Part model, mm, in its own coordinate system. A direction names the side the tool comes from. Round coordinates to 2 decimals unless told otherwise and drop trailing zeros. Loops run counter-clockwise (first coordinate to the right, second up) from the corner with the lowest first, then second, coordinate; pieces in that order, holes last.
(1) Cut at D-D on x = -13.5. List the corners of the cut face in (y, z), then the cut area to 3 significant figures.
(2) Tool access for faces 5 (the face through (-41.03, -29.13, 3.86)), 6 (the face through (23.855, -29.125, 33.602)), 7 (the face through (-32.84, -29.13, -19.32)): list every direction of +Z, -Z, +X, -X, +Y, -Y with a clear straight run to the whole face (end or side of a thin tool).
(3) Cut at C-C on z = 0. List the corners of the cut face in (x, y) (3 decimals), then the cut area to 3 significant figures.
(4) Cut at B-B on y = -31.5. List the corners of the cut face in (x, z), then the cut area to 3 significant figures.
(5) Cut at A-A on x = 0. List the corners of the cut face in (y, z) (3 decimals).
(6) Mould opens along Z. For faces 1 (the face through (-0.3, -29.1, 38.1)), 2 (the face through (41.11, -29.13, 3.9)), 3 (the face through (34, -44.45, -19)), 4 (the face through (12, -14.224, -12)) say: +Z half, -Z half, draft (parallel to the pull), parting line (faces both ways), or undercut.
(7) Probe probe 1 along Z at (x, y) = (0, -5) (3 decimals); probe 2 along Z at (x, y) = (5, -9); probe 3 along Y at (x, z) = (-41.5, -39). List the from-to ranges inside material, lowest first.
(8) Flat gauge pins, fed straight in: pin 1 (5 mm diameter, centred on x = 10.5, y = -28, fed in from -Z); pin 2 (8 mm diameter, centred on y = -33.5, z = -40.5, fed in from +X); pin 3 (10 mm diameter, centred on x = -22.5, y = -30, fed in from -Z). Where does each tip first touch, or does it go through?
from build123d import *

# Parameters (mm, degrees)
F0_R     = 57.15
F1_DEPTH = 14.224
F2_R     = 15.875
F3_DEPTH = 25.4
F4_R     = 7.112
F5_DEPTH = 25.4
F7_DEPTH = 30.226


with BuildPart() as f1:
    # F0 (on Front) → F1 (new body)
    with BuildSketch(Plane.XZ):
        Circle(F0_R)
    extrude(amount=F1_DEPTH)

    # F2 (on face) → F3 (cut)
    with BuildSketch(Plane.XZ.offset(14.224)):
        Circle(F2_R)
    extrude(amount=-F3_DEPTH, mode=Mode.SUBTRACT)

    # F4 (on face) → F5 (cut)
    with BuildSketch(Plane.XZ.offset(14.224)):
        with Locations((0, -38.1)):
            Circle(F4_R)
        with Locations((32.995568, 19.05)):
            Circle(F4_R)
        with Locations((-32.995568, 19.05)):
            Circle(F4_R)
    extrude(amount=-F5_DEPTH, mode=Mode.SUBTRACT)

    # F6 (on face) → F7 (join)
    with BuildSketch(Plane.XZ.offset(14.224)):
        with BuildLine():
            Line((-38.032706, 2.26346), (-44.108679, 5.4979))
            ThreePointArc((-44.108679, 5.4979), (-38.494829, -22.225), (-17.293019, -40.948187))
            Line((-17.293019, -40.948187), (-17.056139, -34.06902))
            ThreePointArc((-17.056139, -34.06902), (-32.995568, -19.05), (-38.032706, 2.26346))
        make_face()
        with BuildLine():
            ThreePointArc((-20.976567, 31.80556), (0, 38.1), (20.976567, 31.80556))
            Line((20.976567, 31.80556), (26.81566, 35.450287))
            ThreePointArc((26.81566, 35.450287), (0, 44.45), (-26.81566, 35.450287))
            Line((-26.81566, 35.450287), (-20.976567, 31.80556))
        make_face()
        with BuildLine():
            Line((17.056139, -34.06902), (17.293019, -40.948187))
            ThreePointArc((17.293019, -40.948187), (38.494829, -22.225), (44.108679, 5.4979))
            Line((44.108679, 5.4979), (38.032706, 2.26346))
            ThreePointArc((38.032706, 2.26346), (32.995568, -19.05), (17.056139, -34.06902))
        make_face()
    extrude(amount=F7_DEPTH)


solid = f1.part
Final values:
1. outline: (-44.45, 35.63) - (-14.22, 35.63) - (-14.22, 8.35) - (0, 8.35) - (0, 55.53) - (-14.22, 55.53) - (-14.22, 42.35) - (-44.45, 42.35) - close; (-14.22, -55.53) - (0, -55.53) - (0, -8.35) - (-14.22, -8.35) - close
1. area: 1,550 mm2
2. face 5: +Z, -Y
2. face 6: +X, -Y
2. face 7: -Y
3. outline: (-57.15, -14.224) - (-44.45, -14.224) - (-44.45, -44.45) - (-38.1, -44.45) - (-38.1, -14.224) - (-15.875, -14.224) - (-15.875, 0) - (-57.15, 0) - close; (15.875, -14.224) - (38.1, -14.224) - (38.1, -44.45) - (44.45, -44.45) - (44.45, -14.224) - (57.15, -14.224) - (57.15, 0) - (15.875, 0) - close
3. area: 1,560 mm2
4. outline: (-44.11, 5.5) arc R44.45 ccw to (-17.29, -40.95) - (-17.06, -34.07) arc R38.1 cw to (-38.03, 2.26) - close; (-26.82, 35.45) - (-20.98, 31.81) arc R38.1 cw to (20.98, 31.81) - (26.82, 35.45) arc R44.45 ccw to start; (17.06, -34.07) - (17.29, -40.95) arc R44.45 ccw to (44.11, 5.5) - (38.03, 2.26) arc R38.1 cw to start
4. area: 972 mm2
5. outline: (-44.45, 38.1) - (-14.224, 38.1) - (-14.224, 15.875) - (0, 15.875) - (0, 57.15) - (-14.224, 57.15) - (-14.224, 44.45) - (-44.45, 44.45) - close; (-14.224, -57.15) - (0, -57.15) - (0, -45.212) - (-14.224, -45.212) - close; (-14.224, -30.988) - (0, -30.988) - (0, -15.875) - (-14.224, -15.875) - close
6. face 1: undercut
6. face 2: +Z half
6. face 3: draft
6. face 4: undercut
7. probe 1: z = -57.15 to -45.212, -30.988 to -15.875, 15.875 to 57.15
7. probe 2: z = -56.93 to -43.16, -33.04 to -15.07, 15.07 to 56.93
7. probe 3: y = -14.22 to 0
8. pin 1: stops at z = 35.81
8. pin 2: stops at x = 25.37
8. pin 3: stops at z = -40.86
